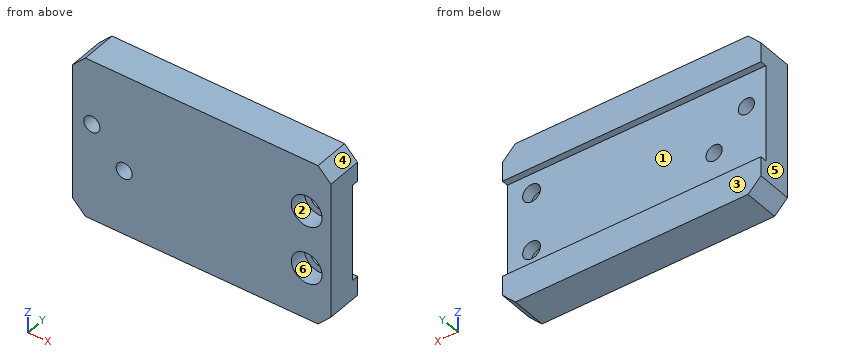
from build123d import *

# Parameters (mm, degrees)
RESSALTO_EXTRUS_O1_DEPTH = 11
ESBO_O2_W                = 80
ESBO_O2_H                = 30
CORTE_EXTRUS_O1_DEPTH    = 2
ESBO_O4_R                = 2.5
CORTE_EXTRUS_O2_DEPTH    = 85.297093663
ESBO_O5_R                = 2.75
CORTE_EXTRUS_O3_DEPTH    = 85.297093663
CHANFRO2_SIZE            = 4
ESBO_O7_R                = 4.75
CORTE_EXTRUS_O6_DEPTH    = 5.4


with BuildPart() as part:
    # Esboço1 → Ressalto-extrusão1 (new body)
    with BuildSketch(Plane(origin=(0, 0, 0), x_dir=(1, 0, 0), z_dir=(0, 1, 0))):
        Polygon((0, 0), (0, -25), (80, -25), (80, 25), (0, 25), align=None)
    extrude(amount=RESSALTO_EXTRUS_O1_DEPTH)

    # Esboço2 → Corte-extrusão1 (cut)
    with BuildSketch(Plane(origin=(0, 11, 0), x_dir=(1, 0, 0), z_dir=(0, 1, 0))):
        with Locations((40, 0)):
            Rectangle(ESBO_O2_W, ESBO_O2_H)
    extrude(amount=-CORTE_EXTRUS_O1_DEPTH, mode=Mode.SUBTRACT)

    # Esboço4 → Corte-extrusão2 (cut, through all)
    with BuildSketch(Plane(origin=(0, 9, 0), x_dir=(1, 0, 0), z_dir=(0, 1, 0))):
        with Locations(Location((16, 5, 0), (0, 0, 270))):
            Circle(ESBO_O4_R)
        with Locations(Location((6, -5, 0), (0, 0, 270))):
            Circle(ESBO_O4_R)
    extrude(amount=-CORTE_EXTRUS_O2_DEPTH, mode=Mode.SUBTRACT)

    # Esboço5 → Corte-extrusão3 (cut, through all)
    with BuildSketch(Plane(origin=(0, 9, 0), x_dir=(1, 0, 0), z_dir=(0, 1, 0))):
        with Locations(Location((72.5, 9, 0), (0, 0, 270))):
            Circle(ESBO_O5_R)
        with Locations(Location((72.5, -9, 0), (0, 0, 270))):
            Circle(ESBO_O5_R)
    extrude(amount=-CORTE_EXTRUS_O3_DEPTH, mode=Mode.SUBTRACT)

    # Chanfro2
    chanfro2_edges = [part.edges().sort_by_distance(p)[0] for p in [
        (0, 5.5, -25),
        (80, 5.5, -25),
        (80, 5.5, 25),
        (0, 5.5, 25),
    ]]
    chamfer(chanfro2_edges, length=CHANFRO2_SIZE)

    # Esboço7 → Corte-extrusão6 (cut)
    with BuildSketch(Plane.XZ):
        with Locations(Location((72.5, 9, 0), (0, 0, 270))):
            Circle(ESBO_O7_R)
        with Locations(Location((72.5, -9, 0), (0, 0, 270))):
            Circle(ESBO_O7_R)
    extrude(amount=-CORTE_EXTRUS_O6_DEPTH, mode=Mode.SUBTRACT)


solid = part.part
Design review of the part built by this model. Coordinates are the model's own, in mm. Face numbers are marked on the shaded views. A direction names the side the tool comes from. Round coordinates to 2 decimals unless told otherwise and drop trailing zeros. Loops run counter-clockwise (first coordinate to the right, second up) from the corner with the lowest first, then second, coordinate; pieces in that order, holes last. Notation, with made-up numbers: (61, -38) - (100, -38) arc R25 cw to (100, -24) - close; hole circle Ø7 at (-38, 71). An arc over 180 degrees is marked (long way). One line per item, written item: value. Start each with the question number.
1) Insertion check: pin 1 Ø7 at (x, z) = (72.5, 9) entering from -Y; pin 2 Ø1.5 at (x, z) = (16, 14) entering from +Y. Each pin has a flat end and moves straight along its axis. Give the tip position at first contact, or say it passes through.
2) For the marked faces 1, 2 and 3, list the 3-axis set-ups (+Z, -Z, +X, -X, +Y, -Y) from which the entire face can be reached by the end or side of a thin tool; tool diameter is ignored.
3) Consider section D-D on x = 72.5. Give the boundary of the cut face in (y, z).
4) Consider section A-A on z = 9. Give the boundary of the cut face in (x, y), then the cut area to 3 significant figures.
5) Consider section C-C on y = 3.5. Give the boundary of the cut face in (x, z).
6) To check wall thickness, follow L1, parallel to X at y = 8.05, z = 9; L2, parallel to X at y = 2.15, z = -9; L3, parallel to Z at x = 46.5, y = 9.5. State the ranges of each line that lie inside material, in increasing order. Write a range as from..to.
7) Draft analysis for pull direction X (two halves, no side actions). For the marked faces 4, 5 and 6, state which applies: +X half, -X half, draft (parallel to the pull), parting line (faces both ways), or undercut.
8) Consider section B-B on x = 16. Give the boundary of the cut face in (y, z).
Reported:
1. pin 1: stops at y = 5.4
1. pin 2: stops at y = 9
2. face 1: +X, -X, +Y
2. face 2: -Y
2. face 3: +Z, -Z, +X, -X, +Y
3. outline: (0, -25) - (11, -25) - (11, -15) - (9, -15) - (9, -11.75) - (5.4, -11.75) - (5.4, -13.75) - (0, -13.75) - close; (0, -4.25) - (5.4, -4.25) - (5.4, -6.25) - (9, -6.25) - (9, 6.25) - (5.4, 6.25) - (5.4, 4.25) - (0, 4.25) - close; (0, 13.75) - (5.4, 13.75) - (5.4, 11.75) - (9, 11.75) - (9, 15) - (11, 15) - (11, 25) - (0, 25) - close
4. outline: (0, 0) - (67.75, 0) - (67.75, 5.4) - (69.75, 5.4) - (69.75, 9) - (0, 9) - close; (75.25, 5.4) - (77.25, 5.4) - (77.25, 0) - (80, 0) - (80, 9) - (75.25, 9) - close
4. area: 649 mm^2
5. outline: (0, -21) - (4, -25) - (76, -25) - (80, -21) - (80, 21) - (76, 25) - (4, 25) - (0, 21) - close; hole circle Ø5 at (6, 5); hole circle Ø5 at (16, -5); hole circle Ø9.5 at (72.5, -9); hole circle Ø9.5 at (72.5, 9)
6. L1: x = 0..69.75, 75.25..80
6. L2: x = 0..67.75, 77.25..80
6. L3: z = -25..-15, 15..25
7. face 4: +X half
7. face 5: -X half
7. face 6: undercut
8. outline: (0, -25) - (11, -25) - (11, -15) - (9, -15) - (9, -7.5) - (0, -7.5) - close; (0, -2.5) - (9, -2.5) - (9, 15) - (11, 15) - (11, 25) - (0, 25) - close
